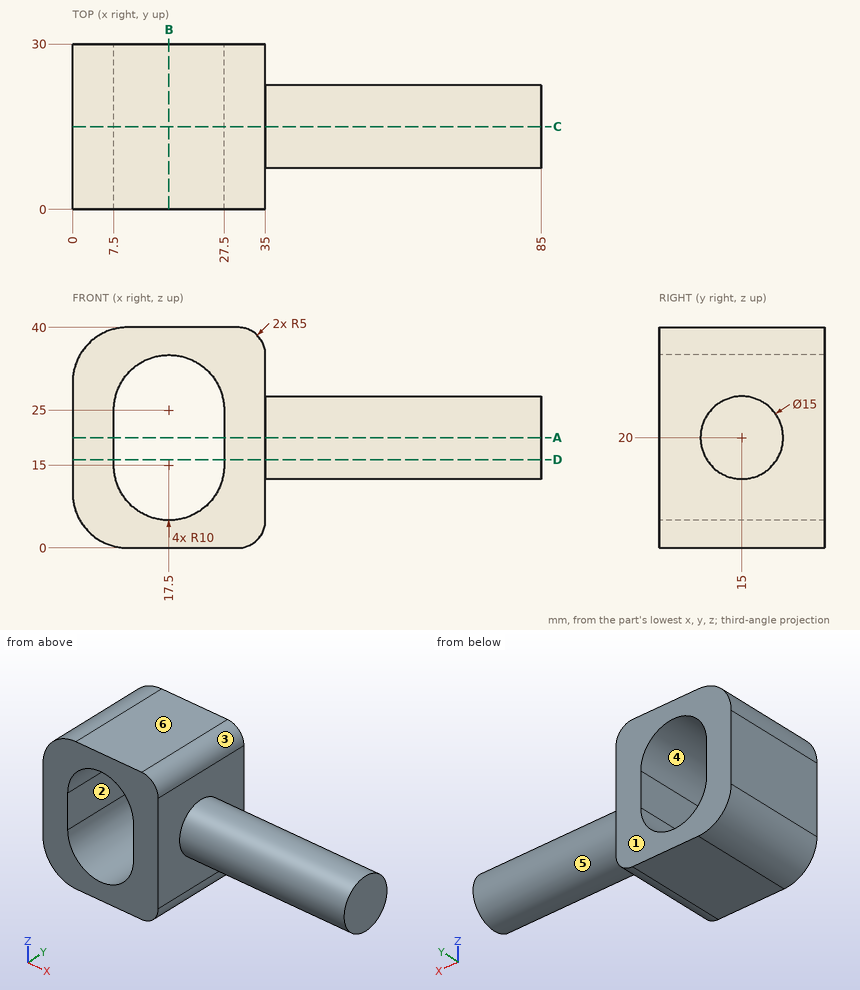
Job drawing, mm, ordinate dimensions from the low corner. One solid piece. A direction names the side the tool comes from. Give positions to 0.01 mm unless a question says otherwise; leave off trailing zeros. Order: outer loops, then holes, each group sorted by start corner. A loop starts at its lowest first (then second) coordinate and runs counter-clockwise, first axis right, second up. Notation, with made-up numbers: M -4.5,8.25 L 28.5,8.25 A31 ccw 28.5,41.25 Z; hole C 25.25,22 d9. An arc over 180 degrees is marked long. Put each result on its own line as item: value. Start each with the question number.
(1) Pull direction X, two halves, no side cores. Call the marked faces 1, 2 and 3: released by +X, released by -X, zero draft, split by the parting line, or undercut.
(2) Drill centre lines: L1, parallel to X at y = 12, z = 14.5; L2, parallel to Z at x = 17, y = 4.5; L3, parallel to X at y = 22.5, z = 16. Where is each one in solid material? Low to high. Write a range as [from, to].
(3) Band-saw the part on A-A on z = 20. Give the cut face in (x, y), then the cut area to 3 significant figures.
(4) Band-saw the part on C-C on y = 15. Give the cut face in (x, z), then the cut area to 3 significant figures.
(5) Pin check, flat tips, straight feed: pin 1 Ø6 at (y, z) = (13.5, 6.5) entering from +X; pin 2 Ø1 at (x, z) = (30.5, 14.5) entering from -Y. Stop position of each tip, or through.
(6) Tool access for the marked faces 4, 5 and 6: list every direction of +Z, -Z, +X, -X, +Y, -Y with a clear straight run to the whole face (end or side of a thin tool).
(7) Band-saw the part on B-B on x = 17.5. Give the cut face in (y, z).
(8) Band-saw the part on D-D on z = 16. Give the cut face in (x, y), then the cut area to 3 significant figures.
Results below:
1. face 1: zero draft
1. face 2: undercut
1. face 3: released by +X
2. L1: x = [0, 7.51], [27.49, 85]
2. L2: z = [0, 5.01], [34.99, 40]
2. L3: x = [0, 7.5], [27.5, 35]
3. outline: M 0,0 L 7.5,0 L 7.5,30 L 0,30 Z; M 27.5,0 L 35,0 L 35,7.5 L 85,7.5 L 85,22.5 L 35,22.5 L 35,30 L 27.5,30 Z
3. area: 1,200 mm2
4. outline: M 0,10 A10 ccw 10,0 L 30,0 A5 ccw 35,5 L 35,12.5 L 85,12.5 L 85,27.5 L 35,27.5 L 35,35 A5 ccw 30,40 L 10,40 A10 ccw 0,30 Z; hole M 7.5,15 A10 ccw 27.5,15 L 27.5,25 A10 ccw 7.5,25 Z
4. area: 1,580 mm2
5. pin 1: stops at x = 35
5. pin 2: stops at y = 0
6. face 4: +Y, -Y
6. face 5: +X
6. face 6: +Z, +X, -X, +Y, -Y
7. outline: M 0,0 L 30,0 L 30,5 L 0,5 Z; M 0,35 L 30,35 L 30,40 L 0,40 Z
8. outline: M 0,0 L 7.5,0 L 7.5,30 L 0,30 Z; M 27.5,0 L 35,0 L 35,8.66 L 85,8.66 L 85,21.34 L 35,21.34 L 35,30 L 27.5,30 Z
8. area: 1,080 mm2
